from build123d import *

# Parameters (mm, degrees)
BOSS_EXTRUDE1_DEPTH = 60
SKETCH2_W           = 101.6
SKETCH2_H           = 25.4
SKETCH2_R           = 2
BOSS_EXTRUDE2_DEPTH = 4.064


with BuildPart() as part:
    # Sketch1 → Boss-Extrude1 (new body)
    with BuildSketch(Plane(origin=(0, 0, 0), x_dir=(1, 0, 0), z_dir=(0, 1, 0))):
        with BuildLine():
            Line((-25.4, -12.7), (25.4, -12.7))
            ThreePointArc((25.4, -12.7), (38.1, 0), (25.4, 12.7))
            Line((25.4, 12.7), (-25.4, 12.7))
            ThreePointArc((-25.4, 12.7), (-38.1, 0), (-25.4, -12.7))
        make_face()
        with BuildLine():
            Line((-25.4, -7.62), (25.4, -7.62))
            ThreePointArc((25.4, -7.62), (33.02, 0), (25.4, 7.62))
            Line((25.4, 7.62), (-25.4, 7.62))
            ThreePointArc((-25.4, 7.62), (-33.02, 0), (-25.4, -7.62))
        make_face(mode=Mode.SUBTRACT)
    extrude(amount=BOSS_EXTRUDE1_DEPTH)

    # Sketch2 → Boss-Extrude2 (add)
    with BuildSketch(Plane.XZ):
        Rectangle(SKETCH2_W, SKETCH2_H)
        with Locations((-44.45, -6.762856744)):
            Circle(SKETCH2_R, mode=Mode.SUBTRACT)
        with Locations((-44.45, 6.762856744)):
            Circle(SKETCH2_R, mode=Mode.SUBTRACT)
        with Locations((44.45, 6.762856744)):
            Circle(SKETCH2_R, mode=Mode.SUBTRACT)
        with Locations((44.45, -6.762856744)):
            Circle(SKETCH2_R, mode=Mode.SUBTRACT)
        with BuildLine():
            Line((-25.4, -7.62), (25.4, -7.62))
            ThreePointArc((25.4, -7.62), (33.02, 0), (25.4, 7.62))
            Line((25.4, 7.62), (-25.4, 7.62))
            ThreePointArc((-25.4, 7.62), (-33.02, 0), (-25.4, -7.62))
        make_face(mode=Mode.SUBTRACT)
    extrude(amount=-BOSS_EXTRUDE2_DEPTH)


solid = part.part
Verification items for the finished model (mm, model axes). A direction names the side the tool comes from. Round coordinates to 2 decimals unless told otherwise and drop trailing zeros. Loops run counter-clockwise (first coordinate to the right, second up) from the corner with the lowest first, then second, coordinate; pieces in that order, holes last. Notation, with made-up numbers: M 44,57 L 78,57 A15 ccw 78,72 Z; hole C -28.5,-28.75 d6. An arc over 180 degrees is marked long. Write each question's results on one line, items separated by ' | '.
1) Section check B-B on x = 44.45. Record the boundary of the cut face in (y, z).
Checks:
outline: M 0,-12.7 L 4.06,-12.7 L 4.06,-8.76 L 0,-8.76 Z; M 0,-4.76 L 4.06,-4.76 L 4.06,4.76 L 0,4.76 Z; M 0,8.76 L 4.06,8.76 L 4.06,12.7 L 0,12.7 Z
2) Gauge pin test, flat ends, axial feed: P1, Ø5, axis at x = 34, y = 53.5, coming from the -Z side; P2, Ø8, axis at y = 51, z = -7.5, coming from the +X side; P3, Ø12, axis at y = 27.5, z = 0.5, coming from the +X side. Record the tip position at first contact, or that the pin passes through.
Checks:
P1: stops at z = -11.14 | P2: stops at x = 37.61 | P3: stops at x = 38.1
3) Section check A-A on z = 0. Record the boundary of the cut face in (x, y).
Checks:
outline: M -50.8,0 L -33.02,0 L -33.02,60 L -38.1,60 L -38.1,4.06 L -50.8,4.06 Z; M 33.02,0 L 50.8,0 L 50.8,4.06 L 38.1,4.06 L 38.1,60 L 33.02,60 Z
4) Access from +Z, -Z, +X, -X, +Y, -Y to the whole of each face (thin tool, end or side, straight path). Record for faces 4 (the cylindrical face through (-38.097, 31.64, -0.279)), 5 (the cylindrical face through (33.02, 29.58, 0.17)), 6 (the cylindrical face through (38.097, 31.64, 0.279)).
Checks:
face 4: -X, +Y | face 5: +Y, -Y | face 6: +X, +Y
5) Section check D-D on x = -20.5. Record the boundary of the cut face in (y, z), then the cut area to 3 significant figures.
Checks:
outline: M 0,-12.7 L 60,-12.7 L 60,-7.62 L 0,-7.62 Z; M 0,7.62 L 60,7.62 L 60,12.7 L 0,12.7 Z | area: 610 mm2
6) Section check C-C on y = 41. Record the boundary of the cut face in (x, z).
Checks:
outline: M -25.4,-12.7 L 25.4,-12.7 A12.7 ccw 25.4,12.7 L -25.4,12.7 A12.7 ccw Z; hole M -25.4,-7.62 L 25.4,-7.62 A7.62 ccw 25.4,7.62 L -25.4,7.62 A7.62 ccw Z
7) Scan lines: L1, parallel to Z at x = -44.45, y = 3.2; L2, parallel to Z at x = 18, y = 31; L3, parallel to Z at x = 44, y = 1. Record each from-to range of solid material in increasing order. Write a range as from..to.
Checks:
L1: z = -12.7..-8.76, -4.76..4.76, 8.76..12.7 | L2: z = -12.7..-7.62, 7.62..12.7 | L3: z = -12.7..-8.71, -4.81..4.81, 8.71..12.7
8) Mould release check, pull along Z, two halves, no side actions. Record for faces 1 (the flat face through (0, 30, -7.62)), 2 (the flat face through (-1, 30, -12.7)), 3 (the flat face through (50.8, 2, 0)): released by +Z, released by -Z, zero draft, split by the parting line, or undercut.
Checks:
face 1: undercut | face 2: released by -Z | face 3: zero draft
